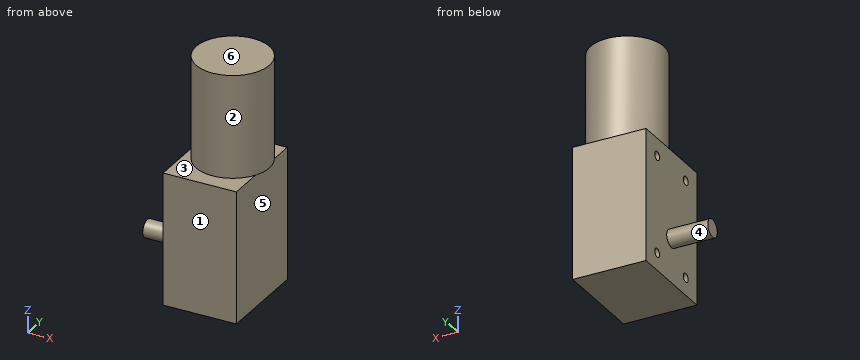
```python
from build123d import *

# Parameters (mm, degrees)
SKETCH1_W           = 45
SKETCH1_H           = 32
BOSS_EXTRUDE1_DEPTH = 25
SKETCH2_R           = 12.5
BOSS_EXTRUDE2_DEPTH = 35
SKETCH3_R           = 3
BOSS_EXTRUDE3_DEPTH = 14
SKETCH4_R           = 1.5
CUT_EXTRUDE1_DEPTH  = 5


with BuildPart() as part:
    # Sketch1 → Boss-Extrude1 (new body)
    with BuildSketch(Plane(origin=(0, 0, 0), x_dir=(0, 0, -1), z_dir=(1, 0, 0))):
        with Locations((-5.67718197, -8.795606883)):
            Rectangle(SKETCH1_W, SKETCH1_H)
    extrude(amount=BOSS_EXTRUDE1_DEPTH)

    # Sketch2 → Boss-Extrude2 (add)
    with BuildSketch(Plane.XY.offset(28.17718197)):
        with Locations(Location((14, -6.795606883, 0), (0, 0, 331.642363424))):
            Circle(SKETCH2_R)
    extrude(amount=BOSS_EXTRUDE2_DEPTH)

    # Sketch3 → Boss-Extrude3 (add)
    with BuildSketch(Plane.ZY):
        with Locations(Location((-1.82281803, -8.795606883, 0), (0, 0, 180))):
            Circle(SKETCH3_R)
    extrude(amount=BOSS_EXTRUDE3_DEPTH)

    # Sketch4 → Cut-Extrude1 (cut)
    with BuildSketch(Plane.ZY):
        with Locations((-10.82281803, 0.204393117)):
            Circle(SKETCH4_R)
        with Locations((22.17718197, 0.204393117)):
            Circle(SKETCH4_R)
        with Locations((22.17718197, -17.795606883)):
            Circle(SKETCH4_R)
        with Locations((-10.82281803, -17.795606883)):
            Circle(SKETCH4_R)
    extrude(amount=-CUT_EXTRUDE1_DEPTH, mode=Mode.SUBTRACT)


solid = part.part
```
Design review of the part built by this model. Coordinates are the model's own, in mm. Face numbers are marked on the shaded views. A direction names the side the tool comes from. Coordinates: 2 decimals unless noted, no trailing zeros. Order: outer loops, then holes, each group sorted by start corner. A loop starts at its lowest first (then second) coordinate and runs counter-clockwise, first axis right, second up.
1) Take a section at B-B, the plane y = -7.5. Give the boundary of the cut face in (x, z).
2) Take a section at A-A, the plane x = 14. Give the boundary of the cut face in (y, z).
3) For the marked faces 4, 5 and 6, list the 3-axis set-ups (+Z, -Z, +X, -X, +Y, -Y) from which the entire face can be reached by the end or side of a thin tool; tool diameter is ignored.
4) Take a section at C-C, the plane z = -6. Give the boundary of the cut face in (x, y), and give its area (3 significant figures).
5) Mouldability with a two-part tool opening along Y and no side actions: class the marked faces 1, 2 and 3 as +Y half, -Y half, draft (parallel to the pull), parting line (faces both ways), or undercut.
6) Wall thickness on line 1 along X through (y, z) = (-16, -5.5); line 2 along Z through (x, y) = (17, -21); line 3 along X through (y, z) = (-9, 1): over which ranges is each line inside the solid? List them lowest first.
7) Clearance check with flat-ended pins moving along their axes: pin 1 (2.5 mm diameter, centred on y = -17.8, z = -10.82, fed in from +X); pin 2 (3.5 mm diameter, centred on y = 0, z = 22, fed in from -X); pin 3 (1 mm diameter, centred on x = 7, z = 39, fed in from -Y); pin 4 (1.6 mm diameter, centred on x = 25.5, y = -5.5, fed in from -Z). State where each tip first meets the part, or that it passes through.
8) Take a section at D-D, the plane z = 44. Give the boundary of the cut face in (x, y), and give its area (3 significant figures).
Returned:
1. outline: (-14, -4.53) - (0, -4.53) - (0, -16.82) - (25, -16.82) - (25, 28.18) - (26.48, 28.18) - (26.48, 63.18) - (1.52, 63.18) - (1.52, 28.18) - (0, 28.18) - (0, 0.88) - (-14, 0.88) - close
2. outline: (-24.8, -16.82) - (7.2, -16.82) - (7.2, 28.18) - (5.7, 28.18) - (5.7, 63.18) - (-19.3, 63.18) - (-19.3, 28.18) - (-24.8, 28.18) - close
3. face 4: -X
3. face 5: -Z, +X, +Y, -Y
3. face 6: +Z, +X, -X, +Y, -Y
4. outline: (0, -24.8) - (25, -24.8) - (25, 7.2) - (0, 7.2) - close
4. area: 800 mm2
5. face 1: -Y half
5. face 2: parting line
5. face 3: draft
6. line 1: x = 0 to 25
6. line 2: z = -16.82 to 28.18
6. line 3: x = -14 to 25
7. pin 1: stops at x = 25
7. pin 2: stops at x = 0
7. pin 3: stops at y = -17.47
7. pin 4: stops at z = -16.82
8. outline: circle Ø25 at (14, -6.8)
8. area: 491 mm2
